Work out the finished part from the listing and answer in its coordinate system (mm). Give positions to 0.01 mm unless a question says otherwise; leave off trailing zeros. Write each loop counter-clockwise with the first axis right and the second up, starting at its lowest first coordinate (ties: lowest second). Pieces come first, ordered by that corner, then holes.
1) Find section A-A (x = 51). Determine the outline of the cut face in (y, z), plus the area to 3 significant figures.
2) Find section B-B (y = 5). Determine the outline of the cut face in (x, z).
3) Straight lines are drawn through the part: probe 1 along Y at (x, z) = (51, 0.5); probe 2 along Y at (x, z) = (-51, 0.9); probe 3 along X at (y, z) = (4.75, 1.45). For each, find the intervals that lie inside material, in ascending order.
Autodesk Inventor part; units mm, degrees
ref_plane "YZ Plane" through (0, 0, 0) normal (1, 0, 0) x (0, 1, 0)
ref_plane "XZ Plane" through (0, 0, 0) normal (0, 1, 0) x (-1, 0, 0)
ref_plane "XY Plane" through (0, 0, 0) normal (0, 0, 1) x (1, 0, 0)
sketch "スケッチ1" plane through (0, 0, 0) normal (0, 0, 1) x (1, 0, 0)
  line L0 (56, 10) -> (-56, 10)
  line L1 (-56, 10) -> (-56, -10)
  line L2 (-56, -10) -> (56, -10)
  line L3 (56, -10) -> (56, 10)
  line L4 (56, 10) -> (-56, -10) construction
  line L5 (-56, 10) -> (56, -10) construction
  point P0 (0, 0)
  dimension "d0" = 112
  dimension "d1" = 20
extrude "押し出し1" add sketch "スケッチ1" along normal blind 1.5
sketch "スケッチ3" plane through (0, 0, 1.5) normal (0, 0, 1) x (1, 0, 0)
  line L0 (56, 10) -> (-56, 10)
  line L1 (-56, 10) -> (-56, -10)
  point P0 (0, 0)
  point P1 (-51, 5)
  point P2 (-51, -5)
  dimension "d10" = 10
  dimension "d11" = 5
  dimension "d12" = 5
hole "穴1" at (-51, 5, 1.5) at (-51, -5, 1.5) direction (0, 0, -1) diameter 3 end through all
sketch "スケッチ5" plane through (0, 0, 1.5) normal (0, 0, 1) x (1, 0, 0)
  point P0 (0, 0)
  point P1 (51, 7)
  point P2 (51, -7)
hole "穴3" at (51, 7, 1.5) at (51, -7, 1.5) direction (0, 0, -1) diameter 2.1 end through all
sketch "スケッチ6" plane through (56, -10, 0) normal (1, 0, 0) x (0, 0, -1)
  line L0 (-1.5, 0) -> (0, 0)
  line L1 (0, 0) -> (0, 20)
  line L2 (0, 20) -> (-1.5, 20)
  line L3 (-1.5, 20) -> (-1.5, 0)
  point P0 (0, 10)
  dimension "d36" = 1.5
  dimension "d37" = 20
extrude "押し出し3" add sketch "スケッチ6" along normal blind 5
properties part number "pre" material "アルミニウム 5052 H32"
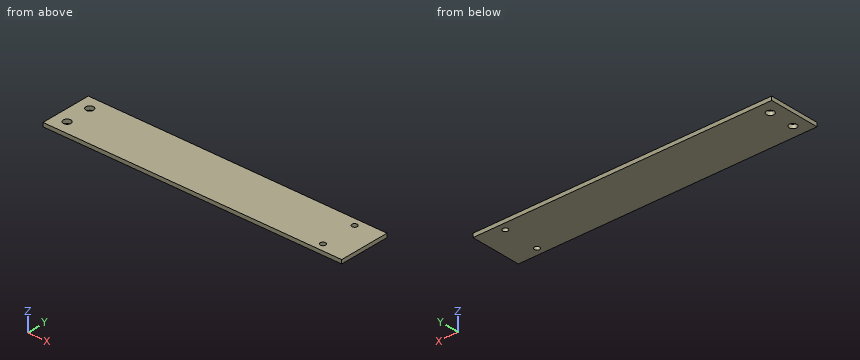
Results:
1. outline: (-10, 0) - (-8.05, 0) - (-8.05, 1.5) - (-10, 1.5) - close; (-5.95, 0) - (5.95, 0) - (5.95, 1.5) - (-5.95, 1.5) - close; (8.05, 0) - (10, 0) - (10, 1.5) - (8.05, 1.5) - close
1. area: 23.7 mm2
2. outline: (-56, 0) - (-52.5, 0) - (-52.5, 1.5) - (-56, 1.5) - close; (-49.5, 0) - (61, 0) - (61, 1.5) - (-49.5, 1.5) - close
3. probe 1: y = -10 to -8.05, -5.95 to 5.95, 8.05 to 10
3. probe 2: y = -10 to -6.5, -3.5 to 3.5, 6.5 to 10
3. probe 3: x = -56 to -52.48, -49.52 to 61
